from build123d import *

# Parameters (mm, degrees)
BOSS_EXTRUDE1_DEPTH = 10
SKETCH3_R           = 2
CUT_EXTRUDE2_DEPTH  = 136


with BuildPart() as part:
    # Sketch1 → Boss-Extrude1 (new body)
    with BuildSketch(Plane.XY):
        Polygon((0, 0), (138, 0), (138, 10), (136, 10), (136, 2), (2, 2), (2, 10), (0, 10), align=None)
    extrude(amount=BOSS_EXTRUDE1_DEPTH)

    # Sketch3 → Cut-Extrude2 (cut)
    with BuildSketch(Plane.ZY):
        with Locations(Location((5, 6, 0), (0, 0, 270))):
            Circle(SKETCH3_R)
    cut_extrude2 = extrude(amount=-CUT_EXTRUDE2_DEPTH, mode=Mode.SUBTRACT)

    # Mirror1: Cut-Extrude2 across plane
    add(cut_extrude2.mirror(Plane.ZY.offset(-69)), mode=Mode.SUBTRACT)


solid = part.part
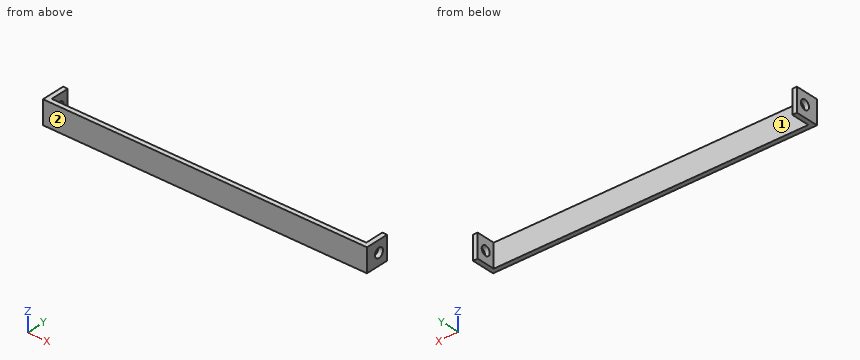
Check sheet for the modelled part. Datum: model origin and axes. Units: mm. Face numbers are marked on the shaded views. Give positions to 0.01 mm unless a question says otherwise; leave off trailing zeros. Order: outer loops, then holes, each group sorted by start corner. A loop starts at its lowest first (then second) coordinate and runs counter-clockwise, first axis right, second up. Notation, with made-up numbers: (54, 43.25) - (87, 43.25) arc R13 ccw to (87, 64.25) - close; hole circle Ø9 at (7, 7). An arc over 180 degrees is marked (long way). Answer as CSV lines item,"result".
1. Scan lines: probe 1 along X at (y, z) = (8.75, 2.75); probe 2 along Z at (x, y) = (1.5, 6); probe 3 along Y at (x, z) = (137, 5). Record each from-to range of solid material in increasing order. Write a range as from..to.
Result sheet:
probe 1,"0..2, 136..138"
probe 2,"0..3, 7..10"
probe 3,"0..4, 8..10"
2. Mould release check, pull along X, two halves, no side actions. Record for the marked faces 1 and 2: released by +X, released by -X, zero draft, split by the parting line, or undercut.
Result sheet:
face 1,"undercut"
face 2,"zero draft"
3. Section check A-A (z = 5). Record the boundary of the cut face in (x, y).
Result sheet:
outline,"(0, 0) - (138, 0) - (138, 4) - (136, 4) - (136, 2) - (2, 2) - (2, 4) - (0, 4) - close; (0, 8) - (2, 8) - (2, 10) - (0, 10) - close; (136, 8) - (138, 8) - (138, 10) - (136, 10) - close"
4. Section check B-B (y = 6). Record the boundary of the cut face in (x, z).
Result sheet:
outline,"(0, 0) - (2, 0) - (2, 3) - (0, 3) - close; (0, 7) - (2, 7) - (2, 10) - (0, 10) - close; (136, 0) - (138, 0) - (138, 3) - (136, 3) - close; (136, 7) - (138, 7) - (138, 10) - (136, 10) - close"
5. Go/stop test with flat-tipped pins: P1, Ø2, axis at x = 75.5, z = 7, coming from the +Y side; P2, Ø4, axis at x = 60, y = 5, coming from the +Z side. Record where each tip stops, or that it passes through.
Result sheet:
P1,"y = 2"
P2,"through"
6. Section check C-C (x = 76.5). Record the boundary of the cut face in (y, z).
Result sheet:
outline,"(0, 0) - (2, 0) - (2, 10) - (0, 10) - close"
